Design review of the part built by this model. Coordinates are the model's own, in mm. Face numbers are marked on the shaded views. A direction names the side the tool comes from. Coordinates: 2 decimals unless noted, no trailing zeros. Loops run counter-clockwise (first coordinate to the right, second up) from the corner with the lowest first, then second, coordinate; pieces in that order, holes last.
Q1. Add section B-B on y = -5. Give the boundary of the cut face in (x, z), and give its area (3 significant figures).
Q2. Add section A-A on z = -22.5. Give the boundary of the cut face in (x, y), and give its area (3 significant figures).
Q3. Machinability: for the marked faces 4, 5 and 6, which of the approach directions +Z, -Z, +X, -X, +Y, -Y give a long, thin tool a straight path to every point of the face, cutting with its end or side? Answer none if there is none.
Q4. Draft analysis for pull direction X (two halves, no side actions). For the marked faces 1, 2 and 3, state which applies: released by +X, released by -X, zero draft, split by the parting line, or undercut.
Q5. For P1, Ø21, axis at x = 61, z = 25, coming from the +Y side; P2, Ø0.9, axis at y = 2, z = -5.5, coming from the +X side; P3, Ø0.9, axis at y = 1.5, z = -14, coming from the -X side, all flat-tipped, find the tip position at first contact; note any pin that passes through.
Q6. Add section C-C on x = -15. Give the boundary of the cut face in (y, z), and give its area (3 significant figures).
Q7. Wall thickness on probe 1 along X at (y, z) = (-5.5, -25); probe 2 along X at (y, z) = (-7.5, 24); probe 3 along X at (y, z) = (-8, 22): over which ranges is each line inside the solid? List them lowest first.
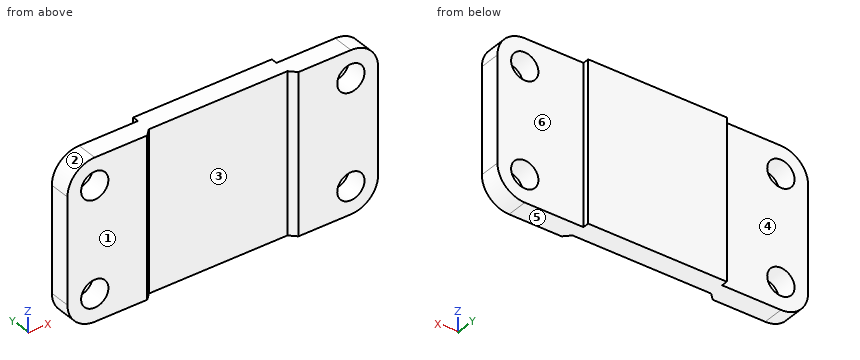
```python
from build123d import *

# Parameters (mm, degrees)
SKETCH1_R           = 6.5
BOSS_EXTRUDE1_DEPTH = 10
CUT_EXTRUDE1_DEPTH  = 107.545764815
SKETCH3_W           = 66
SKETCH3_H           = 3
BOSS_EXTRUDE2_DEPTH = 76


with BuildPart() as part:
    # Sketch1 → Boss-Extrude1 (new body)
    with BuildSketch(Plane(origin=(0, 0, 0), x_dir=(1, 0, 0), z_dir=(0, 1, 0))):
        with BuildLine():
            Line((-61, 38), (61, 38))
            ThreePointArc((61, 38), (70.192388155, 34.192388155), (74, 25))
            Line((74, 25), (74, -25))
            ThreePointArc((74, -25), (70.192388155, -34.192388155), (61, -38))
            Line((61, -38), (-61, -38))
            ThreePointArc((-61, -38), (-70.192388155, -34.192388155), (-74, -25))
            Line((-74, -25), (-74, 25))
            ThreePointArc((-74, 25), (-70.192388155, 34.192388155), (-61, 38))
        make_face()
        with Locations(Location((-61, 25, 0), (0, 0, 270))):
            Circle(SKETCH1_R, mode=Mode.SUBTRACT)
        with Locations(Location((61, 25, 0), (0, 0, 90))):
            Circle(SKETCH1_R, mode=Mode.SUBTRACT)
        with Locations(Location((61, -25, 0), (0, 0, 270))):
            Circle(SKETCH1_R, mode=Mode.SUBTRACT)
        with Locations(Location((-61, -25, 0), (0, 0, 90))):
            Circle(SKETCH1_R, mode=Mode.SUBTRACT)
    extrude(amount=-BOSS_EXTRUDE1_DEPTH)

    # Sketch2 → Cut-Extrude1 (cut, through all)
    with BuildSketch(Plane.XY.offset(38)):
        Polygon((-36, -10), (36, -10), (33, -7), (-33, -7), align=None)
    extrude(amount=-CUT_EXTRUDE1_DEPTH, mode=Mode.SUBTRACT)

    # Sketch3 → Boss-Extrude2 (add, through all)
    with BuildSketch(Plane.XY.offset(38)):
        with Locations((0, 1.5)):
            Rectangle(SKETCH3_W, SKETCH3_H)
    extrude(amount=-BOSS_EXTRUDE2_DEPTH)


solid = part.part
```
Entries:
1. outline: (-74, -25) arc R13 ccw to (-61, -38) - (61, -38) arc R13 ccw to (74, -25) - (74, 25) arc R13 ccw to (61, 38) - (-61, 38) arc R13 ccw to (-74, 25) - close; hole circle Ø13 at (-61, -25); hole circle Ø13 at (-61, 25); hole circle Ø13 at (61, -25); hole circle Ø13 at (61, 25)
1. area: 10,600 mm2
2. outline: (-74, -10) - (-67, -10) - (-67, 0) - (-74, 0) - close; (-55, -10) - (-36, -10) - (-33, -7) - (33, -7) - (36, -10) - (55, -10) - (55, 0) - (33, 0) - (33, 3) - (-33, 3) - (-33, 0) - (-55, 0) - close; (67, -10) - (74, -10) - (74, 0) - (67, 0) - close
2. area: 1,230 mm2
3. face 4: +Z, -Z, -X, +Y
3. face 5: -Z, +X, -X, +Y, -Y
3. face 6: +Z, -Z, +X, +Y
4. face 1: zero draft
4. face 2: released by -X
4. face 3: undercut
5. P1: stops at y = 0
5. P2: stops at x = 33
5. P3: stops at x = -33
6. outline: (-7, -38) - (3, -38) - (3, 38) - (-7, 38) - close
6. area: 760 mm2
7. probe 1: x = -74 to -67.5, -54.5 to 54.5, 67.5 to 74
7. probe 2: x = -74 to -67.42, -54.58 to -33.5, 33.5 to 54.58, 67.42 to 74
7. probe 3: x = -74 to -66.77, -55.23 to -34, 34 to 55.23, 66.77 to 74
